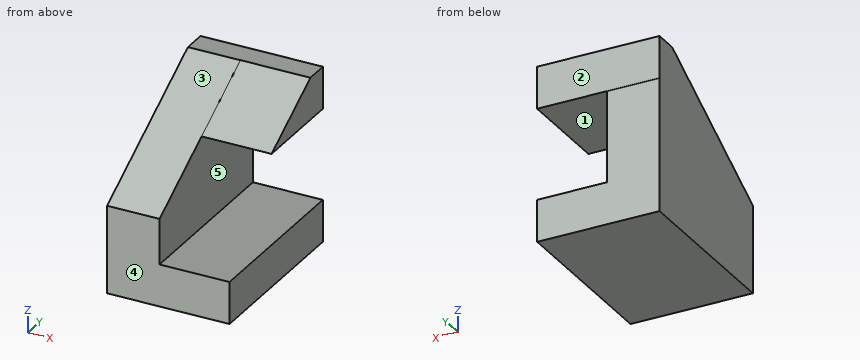
from build123d import *

# Parameters (mm, degrees)
F0_W     = 50
F0_H     = 50
F1_DEPTH = 15
F2_SIZE2 = 43.30127
F2_SIZE  = 25
F4_DEPTH = 35
F5_W     = 50
F5_H     = 12
F6_DEPTH = 35


with BuildPart() as f1:
    # F0 (on Right) → F1 (new body)
    with BuildSketch(Plane.YZ):
        Rectangle(F0_W, F0_H)
    extrude(amount=F1_DEPTH)

    # F2
    f2_edges = [f1.edges().sort_by_distance(p)[0] for p in [
        (7.5, -25, 25),
    ]]
    chamfer(f2_edges, length=F2_SIZE, length2=F2_SIZE2)

    # F3 (on Right) → F4 (join)
    with BuildSketch(Plane.YZ):
        Polygon((-2.48334, 13), (25.0436, 13), (25.0436, 25), (18.3446, 25), align=None)
    extrude(amount=F4_DEPTH)

    # F5 (on Right) → F6 (join)
    with BuildSketch(Plane.YZ):
        with Locations((0, -19)):
            Rectangle(F5_W, F5_H)
    extrude(amount=F6_DEPTH)


solid = f1.part
Input: part model. Units: mm. Frame: model coordinates. Face numbers are marked on the shaded views. A direction names the side the tool comes from. Coordinates: 2 decimals unless noted, no trailing zeros. Order: outer loops, then holes, each group sorted by start corner. A loop starts at its lowest first (then second) coordinate and runs counter-clockwise, first axis right, second up.
1. Access query for the marked faces 4 and 5. Directions: +Z, -Z, +X, -X, +Y, -Y. A direction counts if a zero-diameter tool reaches every point of the face in a straight line with its end or side. Return the directions, or none.
Checked values:
face 4: +Z, -Z, +X, -X, -Y
face 5: +X, +Y, -Y
2. Ray query, line 1 along X through (y, z) = (3, -4); line 2 along Z through (x, y) = (24, -11.5); line 3 along Z through (x, y) = (29.5, 0.5). Return the intervals inside material, ascending.
Checked values:
line 1: x = 0 to 15
line 2: z = -25 to -13
line 3: z = -25 to -13, 13 to 14.72
3. Cut plane D-D, the plane z = -5.5. Return loops of the section in (x, y).
Checked values:
outline: (0, -25) - (15, -25) - (15, 25) - (0, 25) - close
4. Cut plane A-A, the plane x = 33. Return loops of the section in (y, z).
Checked values:
outline: (-25, -25) - (25, -25) - (25, -13) - (-25, -13) - close; (-2.48, 13) - (25.04, 13) - (25.04, 25) - (18.34, 25) - close
5. Cut plane B-B, the plane x = 5.5. Return loops of the section in (y, z).
Checked values:
outline: (-25, -25) - (25, -25) - (25, 13) - (25.04, 13) - (25.04, 25) - (18.3, 25) - (-25, 0) - close
6. Contact query for flat-ended pins moving along their axis: P1, Ø1.5, axis at x = 21, y = -10, coming from the +Z side; P2, Ø2, axis at x = 6.5, z = -15, coming from the +Y side; P3, Ø3, axis at x = 4, z = 18, coming from the -Y side; P4, Ø3, axis at y = -19, z = 5.5, coming from the -X side. Output: stop coordinate, or through.
Checked values:
P1: stops at z = -13
P2: stops at y = 25
P3: stops at y = 3.58
P4: passes through
7. Draft query along Z for the marked faces 1, 2 and 3. Return one class per face: +Z half, -Z half, draft (parallel to the pull), parting line (faces both ways), or undercut.
Checked values:
face 1: undercut
face 2: draft
face 3: +Z half
